```python
from build123d import *

# Parameters (mm, degrees)
BOSS_EXTRUDE1_DEPTH = 25.4
BOSS_EXTRUDE2_DEPTH = 5.08
LPATTERN1_COUNT     = 2
LPATTERN1_PITCH     = 53.34
FILLET7_R           = 2.54
SKETCH4_R           = 1.27
CUT_EXTRUDE1_DEPTH  = 73.186067132


with BuildPart() as part:
    # Sketch1 → Boss-Extrude1 (new, symmetric)
    with BuildSketch(Plane.XY):
        with BuildLine():
            Line((-25.654, 0), (25.654, 0))
            Line((25.654, 0), (25.654, -25.908))
            Line((25.654, -25.908), (23.876, -25.908))
            Line((23.876, -25.908), (23.876, -28.448))
            Line((23.876, -28.448), (29.464, -28.448))
            Line((29.464, -28.448), (29.464, 1.27))
            ThreePointArc((29.464, 1.27), (0, 6.294600126), (-29.464, 1.27))
            Line((-29.464, 1.27), (-29.464, -28.448))
            Line((-29.464, -28.448), (-23.876, -28.448))
            Line((-23.876, -28.448), (-23.876, -25.908))
            Line((-23.876, -25.908), (-25.654, -25.908))
            Line((-25.654, -25.908), (-25.654, 0))
        make_face()
    extrude(amount=BOSS_EXTRUDE1_DEPTH, both=True)

    # Sketch2 → Boss-Extrude2 (add)
    with BuildSketch(Plane.XY.offset(25.4)):
        with BuildLine():
            Line((29.464, -28.448), (29.464, 2.54))
            ThreePointArc((29.464, 2.54), (0, 7.564600126), (-29.464, 2.54))
            Line((-29.464, 2.54), (-29.464, -28.448))
            Line((-29.464, -28.448), (-23.876, -28.448))
            Line((-23.876, -28.448), (-23.876, -25.908))
            Line((-23.876, -25.908), (-25.654, -25.908))
            Line((-25.654, -25.908), (-25.654, 0))
            Line((-25.654, 0), (25.654, 0))
            Line((25.654, 0), (25.654, -25.908))
            Line((25.654, -25.908), (23.876, -25.908))
            Line((23.876, -25.908), (23.876, -28.448))
            Line((23.876, -28.448), (29.464, -28.448))
        make_face()
    boss_extrude2 = extrude(amount=BOSS_EXTRUDE2_DEPTH)

    # LPattern1: Boss-Extrude2 ×2
    with Locations(*[(0, 0, -i * LPATTERN1_PITCH) for i in range(1, LPATTERN1_COUNT)]):
        add(boss_extrude2)

    # Fillet7
    fillet7_edges = [part.edges().sort_by_distance(p)[0] for p in [
        (-29.464, 1.27, 1.27),
        (29.464, 1.27, 1.27),
    ]]
    fillet(fillet7_edges, radius=FILLET7_R)

    # Sketch4 → Cut-Extrude1 (cut, through all)
    with BuildSketch(Plane.ZY.offset(29.464)):
        with Locations((0, -11.938)):
            Circle(SKETCH4_R)
    extrude(amount=-CUT_EXTRUDE1_DEPTH, mode=Mode.SUBTRACT)


solid = part.part
```
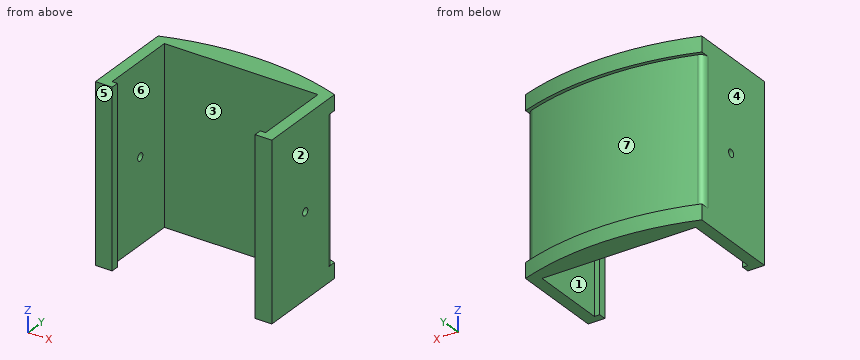
Design review of the part built by this model. Coordinates are the model's own, in mm. Face numbers are marked on the shaded views. A direction names the side the tool comes from. Give positions to 0.01 mm unless a question says otherwise; leave off trailing zeros. Loops run counter-clockwise (first coordinate to the right, second up) from the corner with the lowest first, then second, coordinate; pieces in that order, holes last. Notation, with made-up numbers: (73, 33.25) -> (128, 33.25) arc R23 ccw to (128, 47.25) -> close; hole circle Ø3 at (88.5, 70.5). An arc over 180 degrees is marked (long way). Write each question's results on one line, items separated by ' | '.
Q1. Take a section at B-B, the plane y = -2.5. Write out the cut boundary in (x, z), plus the area to 3 significant figures.
Reply:
outline: (-29.46, -27.94) -> (-25.65, -27.94) -> (-25.65, 30.48) -> (-29.46, 30.48) -> close; (25.65, -27.94) -> (29.46, -27.94) -> (29.46, 30.48) -> (25.65, 30.48) -> close | area: 445 mm²
Q2. Take a section at A-A, the plane z = 0. Write out the cut boundary in (x, y), plus the area to 3 significant figures.
Reply:
outline: (-29.46, -28.45) -> (-23.88, -28.45) -> (-23.88, -25.91) -> (-25.65, -25.91) -> (-25.65, -13.21) -> (-29.46, -13.21) -> close; (-29.46, -10.67) -> (-25.65, -10.67) -> (-25.65, 0) -> (25.65, 0) -> (25.65, -10.67) -> (29.46, -10.67) -> (29.46, -0.55) arc R2.54 ccw to (27.72, 1.86) arc R88.9 ccw to (-27.72, 1.86) arc R2.54 ccw to (-29.46, -0.55) -> close; (23.88, -28.45) -> (29.46, -28.45) -> (29.46, -13.21) -> (25.65, -13.21) -> (25.65, -25.91) -> (23.88, -25.91) -> close | area: 479 mm²
Q3. Take a section at C-C, the plane z = -9.5. Write out the cut boundary in (x, y).
Reply:
outline: (-29.46, -28.45) -> (-23.88, -28.45) -> (-23.88, -25.91) -> (-25.65, -25.91) -> (-25.65, 0) -> (25.65, 0) -> (25.65, -25.91) -> (23.88, -25.91) -> (23.88, -28.45) -> (29.46, -28.45) -> (29.46, -0.55) arc R2.54 ccw to (27.72, 1.86) arc R88.9 ccw to (-27.72, 1.86) arc R2.54 ccw to (-29.46, -0.55) -> close
Q4. The part is to be moulded in two halves that separate along X. For the marked faces 1, 2, 3 and 4, say which applies: +X half, -X half, draft (parallel to the pull), parting line (faces both ways), or undercut.
Reply:
face 1: undercut | face 2: +X half | face 3: undercut | face 4: -X half
Q5. Wall thickness on L1, parallel to Y at x = 25.5, z = -2.5; L2, parallel to X at y = -12.5, z = -12.5; L3, parallel to Y at x = -28.7, z = 0: over which ranges is each line inside the solid? List them lowest first.
Reply:
L1: y = -28.45 to -25.91, 0 to 2.56 | L2: x = -29.46 to -25.65, 25.65 to 29.46 | L3: y = -28.45 to -13.21, -10.67 to 1.27
Q6. Take a section at D-D, the plane x = 9. Write out the cut boundary in (y, z).
Reply:
outline: (0, -27.94) -> (7.11, -27.94) -> (7.11, -22.86) -> (5.84, -22.86) -> (5.84, 25.4) -> (7.11, 25.4) -> (7.11, 30.48) -> (0, 30.48) -> close
Q7. For pin 1 Ø5 at (x, z) = (-5, -11.5) entering from +Y; pin 2 Ø0.5 at (x, z) = (-24.5, -3) entering from +Y; pin 3 Ø3 at (y, z) = (-11.938, 0) entering from +X; pin 4 Ø2 at (x, z) = (7, -11) entering from -Y, all flat-tipped, find the tip position at first contact; note any pin that passes through.
Reply:
pin 1: stops at y = 6.26 | pin 2: stops at y = 2.92 | pin 3: stops at x = 29.46 | pin 4: stops at y = 0
Q8. Machinability: for the marked faces 5, 6 and 7, which of the approach directions +Z, -Z, +X, -X, +Y, -Y give a long, thin tool a straight path to every point of the face, cutting with its end or side? Answer none if there is none.
Reply:
face 5: +Z, -Z, +X, -X, -Y | face 6: +Z, -Z | face 7: +Y
